Can you work these out from the model? Positions are in its coordinate system, mm. A direction names the side the tool comes from. Give positions to 0.01 mm unless a question says otherwise; leave off trailing zeros. Write each loop counter-clockwise with the first axis right and the second up, starting at its lowest first coordinate (ties: lowest second). Pieces come first, ordered by that corner, then holes.
Autodesk Inventor part; units mm, degrees
ref_plane "YZ Plane" through (0, 0, 0) normal (1, 0, 0) x (0, 1, 0)
ref_plane "XZ Plane" through (0, 0, 0) normal (0, 1, 0) x (-1, 0, 0)
ref_plane "XY Plane" through (0, 0, 0) normal (0, 0, 1) x (1, 0, 0)
sketch "Skizze1" plane through (0, 0, 0) normal (0, 1, 0) x (-1, 0, 0)
  circle A0 centre (0, 0) radius 6
  dimension "d0" = 12
extrude "Extrusion1" add sketch "Skizze1" along normal blind 3
sketch "Skizze2" plane through (0, 0, 0) normal (0, -1, 0) x (1, 0, 0)
  circle A0 centre (0, 0) radius 4
  dimension "d3" = 8
extrude "Extrusion2" add sketch "Skizze2" against normal blind 8
sketch "Skizze3" plane through (0, 0, 0) normal (0, -1, 0) x (1, 0, 0)
  circle A0 centre (0, 0) radius 12
  dimension "d6" = 24
extrude "Extrusion3" add sketch "Skizze3" along normal blind 2
sketch "Skizze4" plane through (0, -2, 0) normal (0, -1, 0) x (1, 0, 0)
  point P0 (0, 0)
  point P1 (9, 0)
  dimension "d9" = 9
hole "Bohrung1" at (9, -2, 0) direction (0, 1, 0) diameter 2.4 end through all
pattern_circular "Runde Anordnung1" count 4 over 360 about axis through (0, 0, 0) along (0, -1, 0) of "Bohrung1"
properties part number "dynamixel_pro_frame_shaft"
1) If we mould it in two halves opening along Z, with no side actions, what happens to faces 3 (the face through (6, 1, 0)), 4 (the face through (-0.26, -0.99, 10.17)), 5 (the face through (0, 8, 0))? For each: +Z half, -Z half, draft (parallel to the pull), parting line (faces both ways), or undercut.
Values follow:
face 3: parting line
face 4: undercut
face 5: draft
2) Suppose I cut it at B-B on z = 9. Write out the boundary of the cut face in (x, y).
Values follow:
outline: (-7.94, -2) - (-1.2, -2) - (-1.2, 0) - (-7.94, 0) - close; (1.2, -2) - (7.94, -2) - (7.94, 0) - (1.2, 0) - close
3) Suppose I cut it at A-A on x = -9. Write out the boundary of the cut face in (y, z).
Values follow:
outline: (-2, -7.94) - (0, -7.94) - (0, -1.2) - (-2, -1.2) - close; (-2, 1.2) - (0, 1.2) - (0, 7.94) - (-2, 7.94) - close
4) For faces 1 (the face through (10.17, -0.99, 0.26)), 2 (the face through (1.42, 3, -3.92)), which set-ups out of +Z, -Z, +X, -X, +Y, -Y let a thin tool reach every point of the face, with its end or its side?
Values follow:
face 1: +Y, -Y
face 2: +Y
5) Suppose I cut it at C-C on x = 0. Write out the boundary of the cut face in (y, z), plus the area to 3 significant figures.
Values follow:
outline: (-2, -12) - (0, -12) - (0, -10.2) - (-2, -10.2) - close; (-2, -7.8) - (0, -7.8) - (0, -6) - (3, -6) - (3, -4) - (8, -4) - (8, 4) - (3, 4) - (3, 6) - (0, 6) - (0, 7.8) - (-2, 7.8) - close; (-2, 10.2) - (0, 10.2) - (0, 12) - (-2, 12) - close
area: 114 mm2
6) For pin 1 Ø5 at (y, z) = (-0.5, 7) entering from +X; pin 2 Ø1.5 at (y, z) = (6, 0.5) entering from +X; pin 3 Ø5 at (x, y) = (-6, -0.5) entering from -Z, each with a flat end and sliding along its axis, tell me the tip position at first contact or that it passes through.
Values follow:
pin 1: stops at x = 11.12
pin 2: stops at x = 4
pin 3: stops at z = -11.48
7) Suppose I cut it at D-D on z = 4.5. Write out the boundary of the cut face in (x, y).
Values follow:
outline: (-11.12, -2) - (11.12, -2) - (11.12, 0) - (3.97, 0) - (3.97, 3) - (-3.97, 3) - (-3.97, 0) - (-11.12, 0) - close
8) Please list where these lines run through material, in increasing order: L1, parallel to Z at x = 0, y = -1.6; L2, parallel to Y at x = -8.25, z = -1.5; L3, parallel to Y at x = -3.5, z = 3.5.
Values follow:
L1: z = -12 to -10.2, -7.8 to 7.8, 10.2 to 12
L2: y = -2 to 0
L3: y = -2 to 3
